Check sheet for the modelled part. Datum: model origin and axes. Units: mm. Face numbers are marked on the shaded views. A direction names the side the tool comes from. Round coordinates to 2 decimals unless told otherwise and drop trailing zeros. Loops run counter-clockwise (first coordinate to the right, second up) from the corner with the lowest first, then second, coordinate; pieces in that order, holes last. Notation, with made-up numbers: (-4.75, 80) -> (46.25, 80) arc R19 cw to (46.25, 85) -> close; hole circle Ø11 at (28, -18). An arc over 180 degrees is marked (long way). One line per item, written item: value. Start each with the question number.
1. Cross-section at B-B on x = -15. Record the cut outline in (y, z), then the cut area to 3 significant figures.
2. Cross-section at A-A on y = 22.5. Record the cut outline in (x, z).
3. Go/stop test with flat-tipped pins: pin 1 (20 mm diameter, centred on x = -20.5, y = -16.5, fed in from -Z); pin 2 (0.9 mm diameter, centred on y = -21.5, z = -22, fed in from -X); pin 3 (10 mm diameter, centred on y = 27.5, z = -9.5, fed in from -X); pin 4 (5 mm diameter, centred on x = -15, y = -22.5, fed in from -Z). Record where each tip stops, or that it passes through.
4. Cross-section at C-C on z = -8.5. Record the cut outline in (x, y).
5. Release check for a two-part mould opening along X. For the marked faces 1, 2 and 3 record: +X half, -X half, draft (parallel to the pull), parting line (faces both ways), or undercut.
6. Material ranges on L1, parallel to Y at x = -15, z = 5; L2, parallel to X at y = -22.5, z = 2.75; L3, parallel to Y at x = -15, z = 16.75, recorded low to high.
7. Cross-section at D-D on z = 11. Record the cut outline in (x, y).
8. Set-up check for the marked faces 4, 5, 6 and 7: record each of +Z, -Z, +X, -X, +Y, -Y from which the full face is reachable in a straight line by a thin tool's end or side.
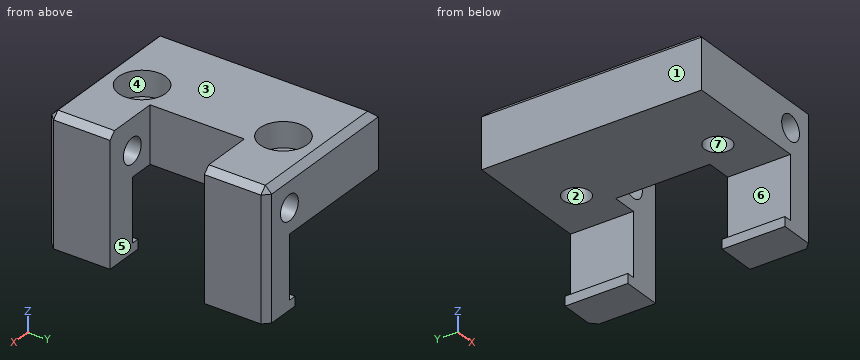
from build123d import *

# Parameters (mm, degrees)
F0_R           = 4
F1_DEPTH       = 35
F3_SIZE        = 2
F2_W           = 18
F2_H           = 41
F4_DEPTH       = 15
F6_D           = 8.4
F6_CBORE_D     = 15
F6_CBORE_DEPTH = 8


# Not quite as in the source:
# - a pattern or mirror of a feature is missing from the dataset's text; its kind, count and spacing are read off the source's solid


with BuildPart() as f1:
    # F0 (on Front) → F1 (new body, symmetric)
    with BuildSketch(Plane.XZ):
        Polygon((-40, 0), (0, 0), (0, -20), (-2.5, -20), (-2.5, -23), (10, -23), (10, 18), (-40, 18), align=None)
        with Locations((0, 8)):
            Circle(F0_R, mode=Mode.SUBTRACT)
    extrude(amount=F1_DEPTH, both=True)

    # F3
    f3_edges = [f1.edges().sort_by_distance(p)[0] for p in [
        (10, 0, 18),
        (10, -35, -2.5),
        (10, 35, -2.5),
        (-15, 35, 18),
        (-15, -35, 18),
        (-40, 0, 18),
    ]]
    chamfer(f3_edges, length=F3_SIZE)

    # F2 (on Front) → F4 (cut, symmetric)
    with BuildSketch(Plane.XZ):
        with Locations((1, -2.5)):
            Rectangle(F2_W, F2_H)
    extrude(amount=F4_DEPTH, both=True, mode=Mode.SUBTRACT)

    # F6 (through all)
    with Locations(Plane.XY.offset(18)):
        with Locations((-15, 22.5)):
            f6 = CounterBoreHole(F6_D / 2, F6_CBORE_D / 2, F6_CBORE_DEPTH)

    # F6_copies: F6 across plane
    add(f6.mirror(Plane(origin=(0, 0, 0), x_dir=(0, 0, -1), z_dir=(0, -1, 0))), mode=Mode.SUBTRACT)


solid = f1.part
Taken from the geometry:
1. outline: (-35, 0) -> (-26.7, 0) -> (-26.7, 10) -> (-30, 10) -> (-30, 18) -> (-33, 18) -> (-35, 16) -> close; (-18.3, 0) -> (18.3, 0) -> (18.3, 10) -> (15, 10) -> (15, 18) -> (-15, 18) -> (-15, 10) -> (-18.3, 10) -> close; (26.7, 0) -> (35, 0) -> (35, 16) -> (33, 18) -> (30, 18) -> (30, 10) -> (26.7, 10) -> close
1. area: 848 mm2
2. outline: (-40, 0) -> (-19.2, 0) -> (-19.2, 10) -> (-22.5, 10) -> (-22.5, 18) -> (-38, 18) -> (-40, 16) -> close; (-10.8, 0) -> (0, 0) -> (0, -20) -> (-2.5, -20) -> (-2.5, -23) -> (10, -23) -> (10, 16) -> (8, 18) -> (-7.5, 18) -> (-7.5, 10) -> (-10.8, 10) -> close; hole circle Ø8 at (0, 8)
3. pin 1: stops at z = 0
3. pin 2: stops at x = -2.5
3. pin 3: stops at x = 0
3. pin 4: passes through
4. outline: (0, -35) -> (8, -35) -> (10, -33) -> (10, -15) -> (0, -15) -> close; (0, 15) -> (10, 15) -> (10, 33) -> (8, 35) -> (0, 35) -> close
5. face 1: -X half
5. face 2: undercut
5. face 3: draft
6. L1: y = -35 to -26.7, -18.3 to 18.3, 26.7 to 35
6. L2: x = -40 to -19.2, -10.8 to 10
6. L3: y = -34.25 to -30, -15 to 15, 30 to 34.25
7. outline: (-40, -35) -> (-2.65, -35) -> (-2.65, -15) -> (-8, -15) -> (-8, 15) -> (-2.65, 15) -> (-2.65, 35) -> (-40, 35) -> close; (2.65, -35) -> (8, -35) -> (10, -33) -> (10, -15) -> (2.65, -15) -> close; (2.65, 15) -> (10, 15) -> (10, 33) -> (8, 35) -> (2.65, 35) -> close; hole circle Ø15 at (-15, -22.5); hole circle Ø15 at (-15, 22.5)
8. face 4: +Z
8. face 5: +Z, -Z, +X
8. face 6: -X, +Y, -Y
8. face 7: +Z, -Z
